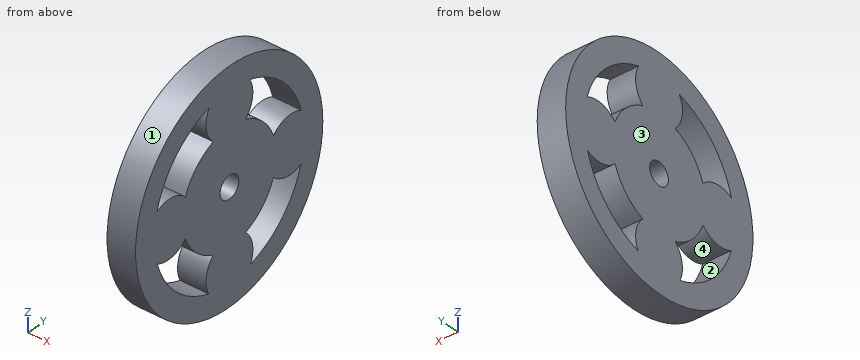
from build123d import *

# Parameters (mm, degrees)
BOX006_W                = 10
BOX006_H                = 45
BOX006_DEPTH            = 45
BOX004_W                = 10
BOX004_H                = 45
BOX004_DEPTH            = 45
CYLINDER012_R           = 5
CYLINDER012_DEPTH       = 10
CYLINDER012_PITCH_ANGLE = 90
SKETCH005_R             = 20
SKETCH005_R_2           = 16
PAD010_DEPTH            = 5
CYLINDER014_R           = 5
CYLINDER014_DEPTH       = 10
CYLINDER014_PITCH_ANGLE = 90
CYLINDER016_R           = 5
CYLINDER016_DEPTH       = 10
CYLINDER016_PITCH_ANGLE = 90
CYLINDER015_R           = 5
CYLINDER015_DEPTH       = 10
CYLINDER015_PITCH_ANGLE = 90
CYLINDER013_R           = 2
CYLINDER013_DEPTH       = 30
CYLINDER013_PITCH_ANGLE = 90
CYLINDER017_R           = 10
CYLINDER017_DEPTH       = 10
CYLINDER017_PITCH_ANGLE = 90


with BuildPart() as cube006:
    # Box006 → Box006 (new body)
    with BuildSketch(Plane(origin=(-10, -54, -57), x_dir=(1, 0, 0), z_dir=(0, 0, 1))):
        with Locations((5, 22.5)):
            Rectangle(BOX006_W, BOX006_H)
    extrude(amount=BOX006_DEPTH)


with BuildPart() as cube004:
    # Box004 → Box004 (new body)
    with BuildSketch(Plane(origin=(5, -54, -57), x_dir=(1, 0, 0), z_dir=(0, 0, 1))):
        with Locations((5, 22.5)):
            Rectangle(BOX004_W, BOX004_H)
    extrude(amount=BOX004_DEPTH)


with BuildPart() as cylinder:
    # Cylinder012 → Cylinder012 (new body)
    with BuildSketch(Plane.XY):
        Circle(CYLINDER012_R)
    extrude(amount=CYLINDER012_DEPTH)


with BuildPart() as cylinder_1:
    # Cylinder012 pitch: moved
    add(cylinder.part.rotate(Axis((0, 0, 0), (0, 1, 0)), CYLINDER012_PITCH_ANGLE))


with BuildPart() as cylinder_2:
    # Cylinder012 placement: moved
    add(cylinder_1.part.moved(Location((-2, -30.5, -21.5))))


with BuildPart() as fusion012:
    # Sketch005 → Pad010 (new body)
    with BuildSketch(Plane.YZ):
        with Locations((-30.558836, -34.409251)):
            Circle(SKETCH005_R)
        with Locations((-30.558836, -34.409251)):
            Circle(SKETCH005_R_2, mode=Mode.SUBTRACT)
    extrude(amount=PAD010_DEPTH)

    # Fusion012: union Cylinder
    add(cylinder_2.part)


with BuildPart() as fusion013:
    # Cylinder014 → Cylinder014 (new body)
    with BuildSketch(Plane.XY):
        Circle(CYLINDER014_R)
    extrude(amount=CYLINDER014_DEPTH)


with BuildPart() as fusion013_1:
    # Cylinder014 pitch: moved
    add(fusion013.part.rotate(Axis((0, 0, 0), (0, 1, 0)), CYLINDER014_PITCH_ANGLE))


with BuildPart() as fusion013_2:
    # Cylinder014 placement: moved
    add(fusion013_1.part.moved(Location((-2, -43.5, -34.5))))

    # Fusion013: union Fusion012
    add(fusion012.part)


with BuildPart() as fusion014:
    # Cylinder016 → Cylinder016 (new body)
    with BuildSketch(Plane.XY):
        Circle(CYLINDER016_R)
    extrude(amount=CYLINDER016_DEPTH)


with BuildPart() as fusion014_1:
    # Cylinder016 pitch: moved
    add(fusion014.part.rotate(Axis((0, 0, 0), (0, 1, 0)), CYLINDER016_PITCH_ANGLE))


with BuildPart() as fusion014_2:
    # Cylinder016 placement: moved
    add(fusion014_1.part.moved(Location((-2, -30.5, -47.5))))

    # Fusion014: union Fusion013
    add(fusion013_2.part)


with BuildPart() as fusion015:
    # Cylinder015 → Cylinder015 (new body)
    with BuildSketch(Plane.XY):
        Circle(CYLINDER015_R)
    extrude(amount=CYLINDER015_DEPTH)


with BuildPart() as fusion015_1:
    # Cylinder015 pitch: moved
    add(fusion015.part.rotate(Axis((0, 0, 0), (0, 1, 0)), CYLINDER015_PITCH_ANGLE))


with BuildPart() as fusion015_2:
    # Cylinder015 placement: moved
    add(fusion015_1.part.moved(Location((-3, -17.5, -34.5))))

    # Fusion015: union Fusion014
    add(fusion014_2.part)


with BuildPart() as cylinder011:
    # Cylinder013 → Cylinder013 (new body)
    with BuildSketch(Plane.XY):
        Circle(CYLINDER013_R)
    extrude(amount=CYLINDER013_DEPTH)


with BuildPart() as cylinder011_1:
    # Cylinder013 pitch: moved
    add(cylinder011.part.rotate(Axis((0, 0, 0), (0, 1, 0)), CYLINDER013_PITCH_ANGLE))


with BuildPart() as cylinder011_2:
    # Cylinder013 placement: moved
    add(cylinder011_1.part.moved(Location((-12, -30.5, -34.5))))


with BuildPart() as cut009:
    # Cylinder017 → Cylinder017 (new body)
    with BuildSketch(Plane.XY):
        Circle(CYLINDER017_R)
    extrude(amount=CYLINDER017_DEPTH)


with BuildPart() as cut009_1:
    # Cylinder017 pitch: moved
    add(cut009.part.rotate(Axis((0, 0, 0), (0, 1, 0)), CYLINDER017_PITCH_ANGLE))


with BuildPart() as cut009_2:
    # Cylinder017 placement: moved
    add(cut009_1.part.moved(Location((-2, -30.5, -34.5))))

    # Cut006: cut Cylinder011
    add(cylinder011_2.part, mode=Mode.SUBTRACT)

    # Fusion016: union Fusion015
    add(fusion015_2.part)

    # Cut010: cut Cube004
    add(cube004.part, mode=Mode.SUBTRACT)

    # Cut009: cut Cube006
    add(cube006.part, mode=Mode.SUBTRACT)


with BuildPart() as cut009_3:
    # Cut009 placement: moved
    add(cut009_2.part.moved(Location((-57.5, -10.5, 45.5))))


solid = cut009_3.part
Check sheet for the modelled part. Datum: model origin and axes. Units: mm. Face numbers are marked on the shaded views. Round coordinates to 2 decimals unless told otherwise and drop trailing zeros. Loops run counter-clockwise (first coordinate to the right, second up) from the corner with the lowest first, then second, coordinate; pieces in that order, holes last. Notation, with made-up numbers: (18.5, -21) -> (40.5, -21) arc R31 ccw to (40.5, 9) -> close; hole circle Ø8 at (27, 78.25). An arc over 180 degrees is marked (long way). Put each result on its own line as item: value. Start each with the question number.
1. Gauge pin test, flat ends, axial feed: pin 1 (3 mm diameter, centred on x = -54.5, z = 2, fed in from -Y); pin 2 (1 mm diameter, centred on x = -54.5, y = -36, fed in from +Z); pin 3 (3 mm diameter, centred on x = -56.5, z = 16, fed in from -Y). Record the tip position at first contact, or that the pin passes through.
2. Draft check along Y on the marked faces 1, 2, 3 and 4. Enter one of: +Y half, -Y half, draft (parallel to the pull), parting line (faces both ways), or undercut.
3. Scan lines: probe 1 along Y at (x, z) = (-56.3, 11); probe 2 along Y at (x, z) = (-57.3, 23); probe 3 along Z at (x, y) = (-56.3, -41). Record each from-to range of solid material in increasing order.
4. Section check D-D (y = -41). Enter the section's corners in (x, z).
5. Section check A-A (z = 5.5). Enter the section's corners in (x, y).
6. Section check B-B (y = -47). Enter the section's corners in (x, z), plus the area to 3 significant figures.
7. Section check C-C (x = -56.75). Enter the section's corners in (y, z), plus the area to 3 significant figures.
Findings:
1. pin 1: stops at y = -59.56
1. pin 2: stops at z = 30.56
1. pin 3: stops at y = -60.77
2. face 1: parting line
2. face 2: undercut
2. face 3: draft
2. face 4: undercut
3. probe 1: y = -61.06 to -43, -39 to -21.06
3. probe 2: y = -57.13 to -51.74, -45.9 to -36.1, -30.37 to -24.99
3. probe 3: z = -8.91 to 9, 13 to 31.09
4. outline: (-57.5, -8.91) -> (-52.5, -8.91) -> (-52.5, 9) -> (-57.5, 9) -> close; (-57.5, 13) -> (-52.5, 13) -> (-52.5, 31.09) -> (-57.5, 31.09) -> close
5. outline: (-57.5, -60.26) -> (-52.5, -60.26) -> (-52.5, -56.05) -> (-57.5, -56.05) -> close; (-57.5, -49.35) -> (-52.5, -49.35) -> (-52.5, -32.65) -> (-57.5, -32.65) -> close; (-57.5, -26.07) -> (-52.5, -26.07) -> (-52.5, -21.86) -> (-57.5, -21.86) -> close
6. outline: (-57.5, -8.01) -> (-52.5, -8.01) -> (-52.5, -3.77) -> (-57.5, -3.77) -> close; (-57.5, 3) -> (-52.5, 3) -> (-52.5, 19) -> (-57.5, 19) -> close; (-57.5, 25.95) -> (-52.5, 25.95) -> (-52.5, 30.19) -> (-57.5, 30.19) -> close
6. area: 122 mm^2
7. outline: circle Ø40 at (-41.06, 11.09); hole (-56.48, 15.34) arc R5 cw to (-50.38, 14.45) arc R10 cw to (-44.45, 20.38) arc R5 cw to (-45.32, 26.51) arc R16 ccw to start; hole (-56.42, 6.63) arc R16 ccw to (-45.44, -4.3) arc R5 cw to (-44.45, 1.62) arc R10 cw to (-50.38, 7.55) arc R5 cw to start; hole circle Ø4 at (-41, 11); hole (-37.55, 1.62) arc R5 cw to (-36.54, -4.26) arc R16 ccw to (-25.72, 6.55) arc R5 cw to (-31.62, 7.55) arc R10 cw to start; hole (-37.55, 20.38) arc R10 cw to (-31.62, 14.45) arc R5 cw to (-25.65, 15.42) arc R16 ccw to (-36.65, 26.47) arc R5 cw to start
7. area: 979 mm^2
